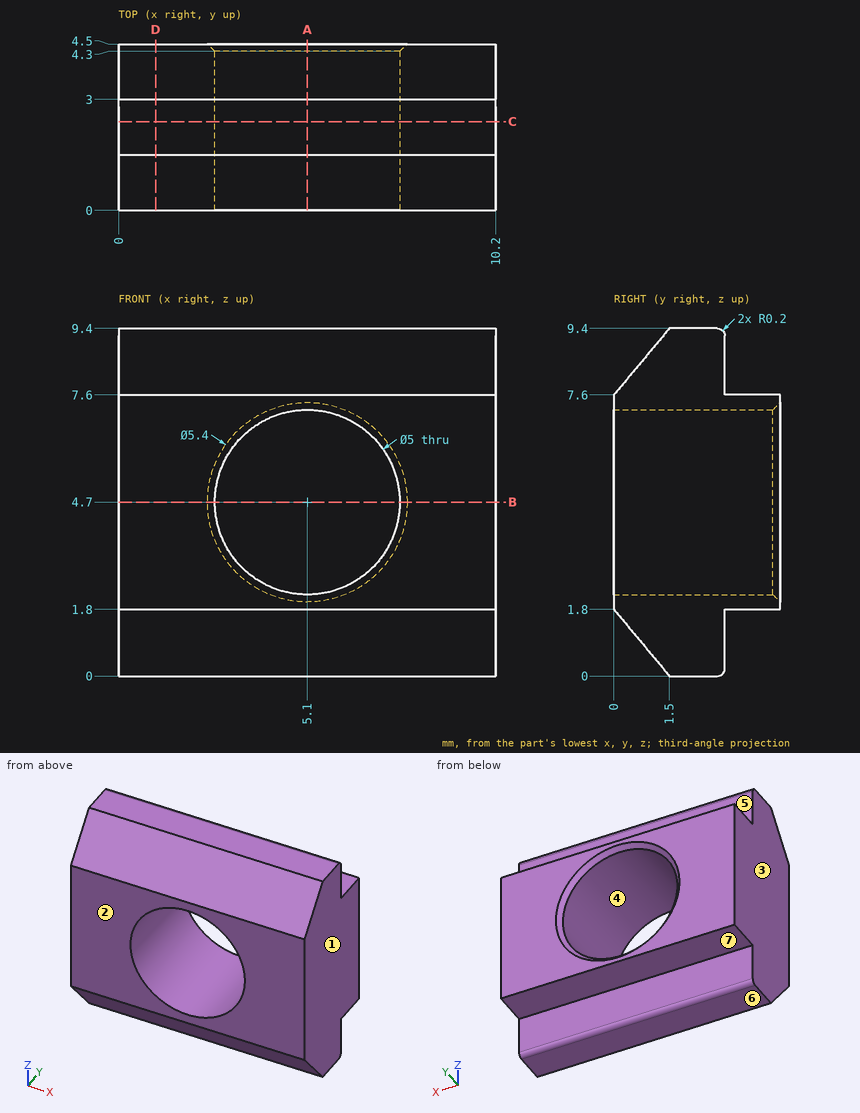
Here's the drawing with two shaded views (mm, measured from the low corner). I have some questions. A direction names the side the tool comes from. Coordinates: 2 decimals unless noted, no trailing zeros. Loops run counter-clockwise (first coordinate to the right, second up) from the corner with the lowest first, then second, coordinate; pieces in that order, holes last. Notation, with made-up numbers: (19, 14) -> (39, 14) arc R27 cw to (39, 53) -> close; hole circle Ø10 at (-29, 82.25). An arc over 180 degrees is marked (long way). Put each result on its own line as item: value. Start each with the question number.
Q1. If I drill on line 1 (Z direction, x = 5.1, y = 2.7); line 2 (X direction, y = 3.4, z = 4.7); line 3 (Z direction, x = 5.1, y = 3.4), over which ranges is the centre line in solid material (lowest first)? Write a range as [from, to].
Q2. For the marked faces 5, 6 and 7, which set-ups out of +Z, -Z, +X, -X, +Y, -Y let a thin tool reach every point of the face, with its end or its side?
Q3. Thinking about a two-plate mould opening in X: for the marked faces 1, 2, 3 and 4, which applies, pulls with the +X half, pulls with the -X half, needs draft (parallel to the pull), parting line crosses it, or undercut?
Q4. I want a section at C-C (y = 2.4). Write out the boundary of the cut face in (x, z), plus the area to 3 significant figures.
Q5. I want a section at D-D (x = 1). Write out the boundary of the cut face in (y, z).
Q6. I'm going to push flat-ended pins straight in: P1, Ø1, axis at x = 5, y = 4, coming from the +Z side; P2, Ø0.5, axis at x = 3, z = 8.5, coming from the +Y side; P3, Ø0.8, axis at x = 3, y = 3.5, coming from the -Z side. Where does each tip first touch, or does it pass through?
Q7. I want a section at A-A (x = 5.1). Write out the boundary of the cut face in (y, z).
Q8. I want a section at B-B (z = 4.7). Write out the boundary of the cut face in (x, y), plus the area to 3 significant figures.
Taken from the geometry:
1. line 1: z = [0, 2.2], [7.2, 9.4]
1. line 2: x = [0, 2.6], [7.6, 10.2]
1. line 3: z = [1.8, 2.2], [7.2, 7.6]
2. face 5: +Z, +X, -X, +Y
2. face 6: -Z, +X, -X, +Y, -Y
2. face 7: -Z, +X, -X, +Y
3. face 1: pulls with the +X half
3. face 2: needs draft
3. face 3: pulls with the -X half
3. face 4: undercut
4. outline: (0, 0) -> (10.2, 0) -> (10.2, 9.4) -> (0, 9.4) -> close; hole circle Ø5 at (5.1, 4.7)
4. area: 76.2 mm2
5. outline: (0, 1.8) -> (1.5, 0) -> (2.8, 0) arc R0.2 ccw to (3, 0.2) -> (3, 1.8) -> (4.5, 1.8) -> (4.5, 7.6) -> (3, 7.6) -> (3, 9.2) arc R0.2 ccw to (2.8, 9.4) -> (1.5, 9.4) -> (0, 7.6) -> close
6. P1: stops at z = 7.6
6. P2: stops at y = 3
6. P3: stops at z = 1.8
7. outline: (0, 1.8) -> (1.5, 0) -> (2.8, 0) arc R0.2 ccw to (3, 0.2) -> (3, 1.8) -> (4.5, 1.8) -> (4.5, 2) -> (4.3, 2.2) -> (0, 2.2) -> close; (0, 7.2) -> (4.3, 7.2) -> (4.5, 7.4) -> (4.5, 7.6) -> (3, 7.6) -> (3, 9.2) arc R0.2 ccw to (2.8, 9.4) -> (1.5, 9.4) -> (0, 7.6) -> close
8. outline: (0, 0) -> (2.6, 0) -> (2.6, 4.3) -> (2.4, 4.5) -> (0, 4.5) -> close; (7.6, 0) -> (10.2, 0) -> (10.2, 4.5) -> (7.8, 4.5) -> (7.6, 4.3) -> close
8. area: 23.4 mm2
